from build123d import *

# Parameters (mm, degrees)
SKETCH1_W            = 103
SKETCH1_H            = 65
BOSS_EXTRUDE1_DEPTH  = 3.25
SKETCH2_W            = 9
SKETCH2_H            = 65
BOSS_EXTRUDE2_DEPTH  = 15
CUT_EXTRUDE1_DEPTH   = 91.985232318
BOSS_EXTRUDE3_DEPTH  = 20
SKETCH5_R            = 1.65
CUT_EXTRUDE2_DEPTH   = 100.891503643
SKETCH11_W           = 103
SKETCH11_H           = 3.25
BOSS_EXTRUDE8_DEPTH  = 5
SKETCH12_W           = 9
SKETCH12_H           = 8
SKETCH12_R           = 1.65
BOSS_EXTRUDE9_DEPTH  = 3.25
SKETCH15_W           = 9
SKETCH15_H           = 3.25
BOSS_EXTRUDE10_DEPTH = 6
FILLET1_R            = 10
FILLET2_R            = 1.5
FILLET3_R            = 3
FILLET4_R            = 3
SKETCH16_W           = 3
SKETCH16_H           = 90
BOSS_EXTRUDE11_DEPTH = 2


# Some blends are built 0.0001 mm under size
with BuildPart() as part:
    # Sketch1 → Boss-Extrude1 (new body)
    with BuildSketch(Plane(origin=(0, 0, 0), x_dir=(1, 0, 0), z_dir=(0, 1, 0))):
        Rectangle(SKETCH1_W, SKETCH1_H)
    extrude(amount=BOSS_EXTRUDE1_DEPTH)

    # Sketch2 → Boss-Extrude2 (add)
    with BuildSketch(Plane(origin=(0, 3.25, 0), x_dir=(1, 0, 0), z_dir=(0, 1, 0))):
        with Locations((-36, 0)):
            Rectangle(SKETCH2_W, SKETCH2_H)
    boss_extrude2 = extrude(amount=BOSS_EXTRUDE2_DEPTH)

    # Sketch3 → Cut-Extrude1 (cut, through all)
    with BuildSketch(Plane(origin=(-31.5, 0, 0), x_dir=(0, 0, -1), z_dir=(1, 0, 0))):
        with BuildLine():
            Line((25.85, 8), (-25.85, 8))
            ThreePointArc((-25.85, 8), (-27.5, 9.65), (-25.85, 11.3))
            Line((-25.85, 11.3), (25.85, 11.3))
            ThreePointArc((25.85, 11.3), (27.5, 9.65), (25.85, 8))
        make_face()
    cut_extrude1 = extrude(amount=-CUT_EXTRUDE1_DEPTH, mode=Mode.SUBTRACT)

    # Sketch4 → Boss-Extrude3 (add)
    with BuildSketch(Plane(origin=(0, 0, -32.5), x_dir=(-1, 0, 0), z_dir=(0, 0, -1))):
        Polygon((51.5, 3.25), (40.5, 3.25), (40.5, 18.25), (31.5, 18.25), (31.5, 3.25), (-51.5, 3.25), (-51.5, 0), (51.5, 0), align=None)
    boss_extrude3 = extrude(amount=BOSS_EXTRUDE3_DEPTH)

    # Sketch5 → Cut-Extrude2 (cut, through all)
    with BuildSketch(Plane(origin=(-31.5, 0, 0), x_dir=(0, 0, -1), z_dir=(1, 0, 0))):
        with Locations((46.339135755, 9.8)):
            Circle(SKETCH5_R)
    cut_extrude2 = extrude(amount=-CUT_EXTRUDE2_DEPTH, mode=Mode.SUBTRACT)

    # Mirror1: Boss-Extrude2, Cut-Extrude1, Boss-Extrude3, Cut-Extrude2 across plane
    add(boss_extrude2.mirror(Plane(origin=(0, 0, 0), x_dir=(0, 0, 1), z_dir=(1, 0, 0))))
    add(cut_extrude1.mirror(Plane(origin=(0, 0, 0), x_dir=(0, 0, 1), z_dir=(1, 0, 0))), mode=Mode.SUBTRACT)
    add(boss_extrude3.mirror(Plane(origin=(0, 0, 0), x_dir=(0, 0, 1), z_dir=(1, 0, 0))))
    add(cut_extrude2.mirror(Plane(origin=(0, 0, 0), x_dir=(0, 0, 1), z_dir=(1, 0, 0))), mode=Mode.SUBTRACT)

    # Sketch11 → Boss-Extrude8 (add)
    with BuildSketch(Plane.XY.offset(32.5)):
        with Locations((0, 1.625)):
            Rectangle(SKETCH11_W, SKETCH11_H)
    extrude(amount=BOSS_EXTRUDE8_DEPTH)

    # Sketch12 → Boss-Extrude9 (add)
    # profile 1 of 4: a face of its own
    with BuildSketch(Plane(origin=(0, 0, 0), x_dir=(1, 0, 0), z_dir=(0, 1, 0))):
        with Locations((56, -36.5)):
            Rectangle(SKETCH12_W, SKETCH12_H)
        with Locations(Location((56, -36.5, 0), (0, 0, 90))):
            Circle(SKETCH12_R, mode=Mode.SUBTRACT)
    # profile 2 of 4: a face of its own
    with BuildSketch(Plane(origin=(0, 0, 0), x_dir=(1, 0, 0), z_dir=(0, 1, 0))):
        with Locations((56, 36.5)):
            Rectangle(SKETCH12_W, SKETCH12_H)
        with Locations(Location((56, 36.5, 0), (0, 0, 90))):
            Circle(SKETCH12_R, mode=Mode.SUBTRACT)
    # profile 3 of 4: a face of its own
    with BuildSketch(Plane(origin=(0, 0, 0), x_dir=(1, 0, 0), z_dir=(0, 1, 0))):
        with Locations((-56, 36.5)):
            Rectangle(SKETCH12_W, SKETCH12_H)
        with Locations(Location((-56, 36.5, 0), (0, 0, 90))):
            Circle(SKETCH12_R, mode=Mode.SUBTRACT)
    # profile 4 of 4: a face of its own
    with BuildSketch(Plane(origin=(0, 0, 0), x_dir=(1, 0, 0), z_dir=(0, 1, 0))):
        with Locations((-56, -36.5)):
            Rectangle(SKETCH12_W, SKETCH12_H)
        with Locations(Location((-56, -36.5, 0), (0, 0, 90))):
            Circle(SKETCH12_R, mode=Mode.SUBTRACT)
    extrude(amount=BOSS_EXTRUDE9_DEPTH)

    # Sketch15 → Boss-Extrude10 (add)
    with BuildSketch(Plane(origin=(0, 0, 32.5), x_dir=(-1, 0, 0), z_dir=(0, 0, -1))):
        with Locations((56, 1.625)):
            Rectangle(SKETCH15_W, SKETCH15_H)
        with Locations((-56, 1.625)):
            Rectangle(SKETCH15_W, SKETCH15_H)
    extrude(amount=BOSS_EXTRUDE10_DEPTH)

    # Fillet1
    # the kernel refuses this fillet: 10 mm, written as the material it adds along each edge
    with BuildSketch(Plane(origin=(51.5, 0, 26.5), x_dir=(1, 0, 0), z_dir=(0, 1, 0)), Plane(origin=(51.5, 0, -40.5), x_dir=(1, 0, 0), z_dir=(0, 1, 0)), Plane(origin=(-51.5, 0, -32.5), x_dir=(-1, 0, 0), z_dir=(0, 1, 0))) as fillet1_piece_1:
        with BuildLine():
            CenterArc((10, 9.949874371), FILLET1_R, 180, 84.260829523)
            Line((0, 9.949874371), (-0.2, 9.949874371))
            Line((-0.2, 9.949874371), (-0.2, 0))
            Line((-0.2, 0), (0, -0.2))
            ThreePointArc((0, -0.2), (4.5, -0.2), (8.98, -0.198997487))
            Line((8.98, -0.198997487), (9, 0))
        make_face()
    extrude(amount=3.25)
    with BuildSketch(Plane(origin=(51.5, 0, -32.5), x_dir=(0, 0, 1), z_dir=(0, 1, 0)), Plane(origin=(-51.5, 0, -40.5), x_dir=(0, 0, -1), z_dir=(0, 1, 0))) as fillet1_piece_2:
        with BuildLine():
            CenterArc((9.949874371, 10), FILLET1_R, 185.739170477, 84.260829523)
            Line((0, 9), (-0.198997487, 8.98))
            ThreePointArc((-0.198997487, 8.98), (-0.2, 4.5), (-0.2, 0))
            Line((-0.2, 0), (0, -0.2))
            Line((0, -0.2), (9.949874371, -0.2))
            Line((9.949874371, -0.2), (9.949874371, 0))
        make_face()
    extrude(amount=3.25)
    with BuildSketch(Plane(origin=(-51.5, 3.25, 26.5), x_dir=(0, 0, -1), z_dir=(0, -1, 0))) as fillet1_piece_3:
        with BuildLine():
            CenterArc((9.949874371, -10), FILLET1_R, 90, 84.260829523)
            Line((0, -9), (-0.198997487, -8.98))
            ThreePointArc((-0.198997487, -8.98), (-0.2, -4.5), (-0.2, 0))
            Line((-0.2, 0), (0, 0.2))
            Line((0, 0.2), (9.949874371, 0.2))
            Line((9.949874371, 0.2), (9.949874371, 0))
        make_face()
    extrude(amount=3.25)

    # Fillet2
    fillet2_edges = [part.edges().sort_by_distance(p)[0] for p in [
        (-51.5, 1.625, 37.5),
        (51.5, 1.625, 37.5),
    ]]
    fillet(fillet2_edges, radius=FILLET2_R)
    fillet2_2_edges = [part.edges().sort_by_distance(p)[0] for p in [
        (-51.5, 1.625, 40.5),
        (51.5, 1.625, 40.5),
    ]]
    fillet(fillet2_2_edges, radius=FILLET2_R - 0.0001)  # a hair under: the kernel refuses the full size

    # Fillet3
    fillet3_edges = [part.edges().sort_by_distance(p)[0] for p in [
        (-60.5, 1.625, 40.5),
        (-60.5, 1.625, -40.5),
        (-60.5, 1.625, -32.5),
        (60.5, 1.625, -40.5),
        (60.5, 1.625, -32.5),
        (60.5, 1.625, 40.5),
        (-60.5, 1.625, 26.5),
        (60.5, 1.625, 26.5),
    ]]
    fillet(fillet3_edges, radius=FILLET3_R)

    # Fillet4
    fillet4_edges = [part.edges().sort_by_distance(p)[0] for p in [
        (-36, 3.25, 32.5),
        (36, 3.25, 32.5),
    ]]
    fillet(fillet4_edges, radius=FILLET4_R)

    # Sketch16 → Boss-Extrude11 (add)
    with BuildSketch(Plane(origin=(0, 3.25, 0), x_dir=(1, 0, 0), z_dir=(0, 1, 0))):
        with Locations((-7, 7.5)):
            Rectangle(SKETCH16_W, SKETCH16_H)
    boss_extrude11 = extrude(amount=BOSS_EXTRUDE11_DEPTH)

    # Mirror2: Boss-Extrude11 across plane
    add(boss_extrude11.mirror(Plane(origin=(0, 0, 0), x_dir=(0, 0, 1), z_dir=(1, 0, 0))))


solid = part.part
Geometry check sheet. Reference: the model listing, model coordinates, mm. A direction names the side the tool comes from. Coordinates: 2 decimals unless noted, no trailing zeros. Order: outer loops, then holes, each group sorted by start corner. A loop starts at its lowest first (then second) coordinate and runs counter-clockwise, first axis right, second up. Notation, with made-up numbers: (7.5, 52.5) -> (13.5, 52.5) arc R17 ccw to (13.5, 63.5) -> close; hole circle Ø6 at (83, -37). An arc over 180 degrees is marked (long way). Use a Markdown table: item, result. Add a question column.
1. Cross-section at B-B (y = 15.75). Enter the section's corners in (x, z), and give its area (3 significant figures).
2. Material ranges on L1, parallel to X at y = 1.95, z = 36.5; L2, parallel to X at y = 7, z = -39.5; L3, parallel to Z at x = -56, y = 2.5, recorded low to high.
3. Go/stop test with flat-tipped pins: pin 1 Ø2 at (x, z) = (-56, -36.5) entering from +Y; pin 2 Ø0.9 at (x, z) = (-6.5, -22) entering from +Y; pin 3 Ø2.5 at (y, z) = (1.5, -51.5) entering from +X; pin 4 Ø5 at (y, z) = (13, -19.5) entering from -X. Record where each tip stops, or that it passes through.
4. Cross-section at C-C (x = 56). Enter the section's corners in (y, z).
5. Cross-section at D-D (z = 2). Enter the section's corners in (x, y).
6. Mould release check, pull along Z, two halves, no side actions. Record for faces 4 (the face through (-59.6, 1.65, 39.64)), 5 (the face through (40.5, 12, -8)), 6 (the face through (53.466, 1.602, -28.505)): pulls with the +Z half, pulls with the -Z half, needs draft (parallel to the pull), parting line crosses it, or undercut.
7. Set-up check for faces 1 (the face through (-36, 12, 32.5)), 2 (the face through (53.36, 1.6, 22.36)), 3 (the face through (-36, 11.3, 0)): record each of +Z, -Z, +X, -X, +Y, -Y from which the full face is reachable in a straight line by a thin tool's end or side.
8. Cross-section at A-A (z = -36.5). Enter the section's corners in (x, y), and give its area (3 significant figures).
Filled sheet:
| question | item | result |
|---|---|---|
| 1 | outline | (-40.5, -52.5) -> (-31.5, -52.5) -> (-31.5, 32.5) -> (-40.5, 32.5) -> close; (31.5, -52.5) -> (40.5, -52.5) -> (40.5, 32.5) -> (31.5, 32.5) -> close |
| 1 | area | 1,530 mm2 |
| 2 | L1 | -60.5 to -57.65, -54.35 to 54.35, 57.65 to 60.5 |
| 2 | L2 | -40.5 to -31.5, 31.5 to 40.5 |
| 2 | L3 | -42.1 to -38.15, -34.85 to -30.9, 24.9 to 34.85, 38.15 to 40.5 |
| 3 | pin 1 | through |
| 3 | pin 2 | y = 5.25 |
| 3 | pin 3 | x = 51.5 |
| 3 | pin 4 | x = -40.5 |
| 4 | outline | (0, -42.1) -> (3.25, -42.1) -> (3.25, -38.15) -> (0, -38.15) -> close; (0, -34.85) -> (3.25, -34.85) -> (3.25, -30.9) -> (0, -30.9) -> close; (0, 24.9) -> (3.25, 24.9) -> (3.25, 34.85) -> (0, 34.85) -> close; (0, 38.15) -> (3.25, 38.15) -> (3.25, 40.5) -> (0, 40.5) -> close |
| 5 | outline | (-51.5, 0) -> (51.5, 0) -> (51.5, 3.25) -> (40.5, 3.25) -> (40.5, 8) -> (31.5, 8) -> (31.5, 3.25) -> (8.5, 3.25) -> (8.5, 5.25) -> (5.5, 5.25) -> (5.5, 3.25) -> (-5.5, 3.25) -> (-5.5, 5.25) -> (-8.5, 5.25) -> (-8.5, 3.25) -> (-31.5, 3.25) -> (-31.5, 8) -> (-40.5, 8) -> (-40.5, 3.25) -> (-51.5, 3.25) -> close; (-40.5, 11.3) -> (-31.5, 11.3) -> (-31.5, 18.25) -> (-40.5, 18.25) -> close; (31.5, 11.3) -> (40.5, 11.3) -> (40.5, 18.25) -> (31.5, 18.25) -> close |
| 6 | face 4 | pulls with the +Z half |
| 6 | face 5 | needs draft |
| 6 | face 6 | undercut |
| 7 | face 1 | +Z, +X, -X, +Y |
| 7 | face 2 | +X, +Y, -Y |
| 7 | face 3 | +X, -X |
| 8 | outline | (-60.5, 0) -> (-57.65, 0) -> (-57.65, 3.25) -> (-60.5, 3.25) -> close; (-54.35, 0) -> (54.35, 0) -> (54.35, 3.25) -> (40.5, 3.25) -> (40.5, 18.25) -> (31.5, 18.25) -> (31.5, 3.25) -> (8.5, 3.25) -> (8.5, 5.25) -> (5.5, 5.25) -> (5.5, 3.25) -> (-5.5, 3.25) -> (-5.5, 5.25) -> (-8.5, 5.25) -> (-8.5, 3.25) -> (-31.5, 3.25) -> (-31.5, 18.25) -> (-40.5, 18.25) -> (-40.5, 3.25) -> (-54.35, 3.25) -> close; (57.65, 0) -> (60.5, 0) -> (60.5, 3.25) -> (57.65, 3.25) -> close |
| 8 | area | 654 mm2 |
